Design review of the part built by this model. Coordinates are the model's own, in mm. Coordinates: 2 decimals unless noted, no trailing zeros. Write each loop counter-clockwise with the first axis right and the second up, starting at its lowest first coordinate (ties: lowest second). Pieces come first, ordered by that corner, then holes.
Q1. Take a section at A-A, the plane z = 1. Write out the cut boundary in (x, y) (3 decimals), plus the area to 3 significant figures.
Q2. For pin 1 Ø1.5 at (y, z) = (-5, 3) entering from +X; pin 2 Ø1.5 at (x, y) = (3, 19) entering from -Z, all flat-tipped, find the tip position at first contact; note any pin that passes through.
Q3. Take a section at C-C, the plane y = -0.5. Write out the cut boundary in (x, z).
Q4. For L1, parallel to Y at x = -5.5, z = 5; L2, parallel to Y at x = -2.5, z = 5.75; L3, parallel to X at y = -7, z = 5, list the stretches that pass through material, from the lowest coordinate up.
Q5. Take a section at B-B, the plane x = 2.75. Write out the cut boundary in (y, z), plus the area to 3 significant figures.
from build123d import *

# Parameters (mm, degrees)
BOSS_EXTRUDE1_DEPTH = 6.35
SKETCH2_W           = 19.05
SKETCH2_H           = 25.4
BOSS_EXTRUDE2_DEPTH = 6.35


with BuildPart() as part:
    # Sketch1 → Boss-Extrude1 (new body)
    with BuildSketch(Plane.XY):
        with BuildLine():
            Line((-9.525, 0), (9.525, 0))
            Line((9.525, 0), (5.861538462, -8.792307692))
            ThreePointArc((5.861538462, -8.792307692), (0, -12.7), (-5.861538462, -8.792307692))
            Line((-5.861538462, -8.792307692), (-9.525, 0))
        make_face()
    extrude(amount=BOSS_EXTRUDE1_DEPTH)

    # Sketch2 → Boss-Extrude2 (add)
    with BuildSketch(Plane.XY.offset(6.35)):
        with Locations((0, 12.7)):
            Rectangle(SKETCH2_W, SKETCH2_H)
    extrude(amount=-BOSS_EXTRUDE2_DEPTH)


solid = part.part
Responses:
1. outline: (-9.525, 0) - (-5.862, -8.792) arc R6.35 ccw to (5.862, -8.792) - (9.525, 0) - (9.525, 25.4) - (-9.525, 25.4) - close
1. area: 652 mm2
2. pin 1: stops at x = 7.75
2. pin 2: stops at z = 0
3. outline: (-9.32, 0) - (9.32, 0) - (9.32, 6.35) - (-9.32, 6.35) - close
4. L1: y = -9.52 to 25.4
4. L2: y = -12.19 to 25.4
4. L3: x = -6.61 to 6.61
5. outline: (-12.07, 0) - (25.4, 0) - (25.4, 6.35) - (-12.07, 6.35) - close
5. area: 238 mm2
